Model file for the job. Use its own axes, mm. Coordinates: 2 decimals unless noted, no trailing zeros. Write each loop counter-clockwise with the first axis right and the second up, starting at its lowest first coordinate (ties: lowest second). Pieces come first, ordered by that corner, then holes. Notation, with made-up numbers: (-20.5, 37.5) -> (16.5, 37.5) arc R20 ccw to (16.5, 44.5) -> close; hole circle Ø10 at (59, -17). An arc over 180 degrees is marked (long way). Answer as a JSON object with one key per item and string values. Group by question number.
from build123d import *

# Parameters (mm, degrees)
BASE_FLANGE2_DEPTH    = 0.7
F_6_CLEARANCE_HOLE1_D = 3.7973
FILLET1_R             = 2


# Sheet-metal steps are written as plain solids
with BuildPart() as part:
    # Sketch1 → Base-Flange2 (new body)
    with BuildSketch(Plane(origin=(0, 0, 0), x_dir=(1, 0, 0), z_dir=(0, 1, 0))):
        Polygon((0, 0), (0, 23), (14.142135624, 37.142135624), (7.071067812, 44.213203436), (-7.071067812, 30.071067812), (-7.071067812, 7.071067812), (-21.213203436, -7.071067812), (-14.142135624, -14.142135624), align=None)
    extrude(amount=-BASE_FLANGE2_DEPTH)

    # #6 Clearance Hole1 (through all)
    with Locations(Plane(origin=(0, 0, 0), x_dir=(1, 0, 0), z_dir=(0, 1, 0))):
        with Locations((-14.139821541, -7.073381895), (-7.068753729, -0.002314083), (1.237436867, 29.653874811), (8.308504679, 36.724942623)):
            Hole(F_6_CLEARANCE_HOLE1_D / 2)

    # Fillet1
    fillet1_edges = [part.edges().sort_by_distance(p)[0] for p in [
        (-14.142135624, -0.35, 14.142135624),
        (-21.213203436, -0.35, 7.071067812),
        (-7.071067812, -0.35, -7.071067812),
        (-7.071067812, -0.35, -30.071067812),
        (7.071067812, -0.35, -44.213203436),
        (14.142135624, -0.35, -37.142135624),
        (0, -0.35, -23),
        (0, -0.35, 0),
    ]]
    fillet(fillet1_edges, radius=FILLET1_R)


solid = part.part
(1) Cut at D-D on z = -26. List the corners of the cut face in (x, y), plus the area to 3 significant figures.
(2) Pull direction Z, two halves, no side cores. Call faces 1 (the face through (1.485, -0.355, -31.536)), 2 (the face through (-17.707, -0.345, 10.577)), 3 (the face through (-4, -0.7, -15)), 4 (the face through (-12.243, -0.355, 6.99)): released by +Z, released by -Z, zero draft, split by the parting line, or undercut.
(3) Wall check: probe 1 along X at (y, z) = (-0.35, -12.5); probe 2 along Z at (x, y) = (-7.5, -0.4); probe 3 along Z at (x, y) = (0.5, -0.2). Give the ranges that are in metal, low to high.
(4) Cut at C-C on y = -0.3. List the corners of the cut face in (x, z).
(5) Cut at A-A on x = 7. List the corners of the cut face in (y, z).
(6) Cut at B-B on z = -37.5. List the corners of the cut face in (x, y), plus the area to 3 significant figures.
Results found:
{
 "1": {"outline": "(-7.07, -0.7) -> (3, -0.7) -> (3, 0) -> (-7.07, 0) -> close", "area": "7.05 mm²"},
 "2": {"face 1": "undercut", "face 2": "released by +Z", "face 3": "zero draft", "face 4": "undercut"},
 "3": {"probe 1": "x = -7.07 to 0", "probe 2": "z = -6.66 to -1.85, 1.85 to 7.5", "probe 3": "z = -37.64 to -31.4, -27.9 to -23.49"},
 "4": {"outline": "(-19.8, 5.66) -> (-7.66, -6.49) arc R2 cw to (-7.07, -7.9) -> (-7.07, -29.24) arc R2 ccw to (-6.49, -30.66) -> (5.66, -42.8) arc R2 ccw to (8.49, -42.8) -> (12.73, -38.56) arc R2 ccw to (12.73, -35.73) -> (0.59, -23.59) arc R2 cw to (0, -22.17) -> (0, -0.83) arc R2 ccw to (-0.59, 0.59) -> (-12.73, 12.73) arc R2 ccw to (-15.56, 12.73) -> (-19.8, 8.49) arc R2 ccw to start; hole circle Ø3.8 at (-14.14, 7.07); hole circle Ø3.8 at (-7.07, 0); hole circle Ø3.8 at (1.24, -29.65); hole circle Ø3.8 at (8.31, -36.72)"},
 "5": {"outline": "(-0.7, -43.38) -> (0, -43.38) -> (0, -38.1) -> (-0.7, -38.1) -> close; (-0.7, -35.35) -> (0, -35.35) -> (0, -30) -> (-0.7, -30) -> close"},
 "6": {"outline": "(0.36, -0.7) -> (6.58, -0.7) -> (6.58, 0) -> (0.36, 0) -> close; (10.04, -0.7) -> (13.28, -0.7) -> (13.28, 0) -> (10.04, 0) -> close", "area": "6.62 mm²"}
}
